Could you check a few things on this model? Use its own coordinates, in mm. Face numbers are marked on the shaded views. Coordinates: 2 decimals unless noted, no trailing zeros. Order: outer loops, then holes, each group sorted by start corner. A loop starts at its lowest first (then second) coordinate and runs counter-clockwise, first axis right, second up. Notation, with made-up numbers: (18.25, 8) -> (29.25, 8) arc R20 cw to (29.25, 38) -> close; hole circle Ø9 at (22, 67.25). An arc over 180 degrees is marked (long way). Put each result on its own line as item: value. Start each with the question number.
Q1. If we section it at A-A (y = -12): Count the separate pieces of the cut face and the enclosed holes in it, and give its area (3 significant figures).
Q2. If we section it at B-B (z = 5.75): Please give me the cut outline in (x, y), and give its area (3 significant figures).
Q3. Please list where these lines run through material, in increasing order: line 1 along Y through (x, z) = (-12, 6); line 2 along X through (y, z) = (-13, 4.5).
Q4. If we section it at C-C (x = -28): Please give me the cut outline in (y, z).
Q5. Will these pins go through, and if not, where does the flat tip stop? pin 1 (1 mm diameter, centred on x = -27, y = 2.5, fed in from -Z); pin 2 (3 mm diameter, centred on x = 24, z = 3.5, fed in from -Y).
Q6. We'd pull the mould along X, two halves only. Please class the marked faces 1, 2, 3 and 4: +X half, -X half, draft (parallel to the pull), parting line (faces both ways), or undercut.
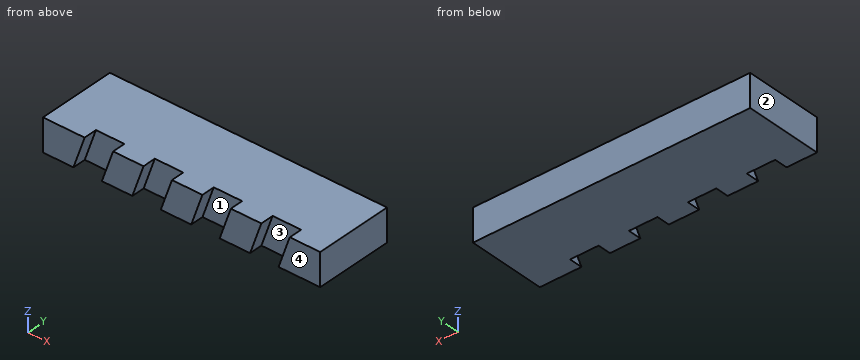
from build123d import *

# Parameters (mm, degrees)
F1_DEPTH = 10
F2_SIZE2 = 3.442485
F2_SIZE  = 9.99999
F3_SIZE2 = 3.442485
F3_SIZE  = 9.99999
F4_SIZE2 = 3.442485
F4_SIZE  = 9.99999
F5_SIZE2 = 3.442485
F5_SIZE  = 9.99999
F6_SIZE2 = 3.442485
F6_SIZE  = 9.99999
F7_SIZE2 = 3.442485
F7_SIZE  = 9.99999
F8_SIZE2 = 3.442485
F8_SIZE  = 9.99999
F9_SIZE2 = 3.442485
F9_SIZE  = 9.99999


# Not quite as in the source:
# - a fillet or chamfer is up to 0.001 mm smaller than in the source, because OpenCascade refuses the exact size


with BuildPart() as f1:
    # F0 (on Top) → F1 (new body)
    with BuildSketch(Plane.XY):
        Polygon((41.1003320895, 9.3217377585), (-44.0996679105, 9.3217377585), (-44.0996679105, -10.6782622415), (-44.0996679105, -14.7482622415), (-31.2996679105, -14.7482622415), (-31.2996679105, -10.6782622415), (-25.9996679105, -10.6782622415), (-25.9996679105, -14.7482622415), (-13.1996679105, -14.7482622415), (-13.1996679105, -10.6782622415), (-7.8996679105, -10.6782622415), (-7.8996679105, -14.7482622415), (4.9003320895, -14.7482622415), (4.9003320895, -10.6782622415), (10.2003320895, -10.6782622415), (10.2003320895, -14.7482622415), (23.0003320895, -14.7482622415), (23.0003320895, -10.6782622415), (28.3003320895, -10.6782622415), (28.3003320895, -14.7482622415), (41.1003320895, -14.7482622415), (41.1003320895, -10.6782622415), align=None)
    extrude(amount=F1_DEPTH)

    # F2 (size 10 and 3.4424952484 in the source; OpenCascade refuses exactly that, so slightly less here)
    f2_edges = [f1.edges().sort_by_distance(p)[0] for p in [
        (-31.299668, -12.713262, 0),
    ]]
    f2_side = f1.faces().sort_by_distance((-31.299668, -12.713262, 5))[0]
    chamfer(f2_edges, length=F2_SIZE, length2=F2_SIZE2, reference=f2_side)

    # F3 (size 10 and 3.4424952484 in the source; OpenCascade refuses exactly that, so slightly less here)
    f3_edges = [f1.edges().sort_by_distance(p)[0] for p in [
        (-25.999668, -12.713262, 10),
    ]]
    f3_side = f1.faces().sort_by_distance((-25.999668, -12.713262, 5))[0]
    chamfer(f3_edges, length=F3_SIZE, length2=F3_SIZE2, reference=f3_side)

    # F4 (size 10 and 3.4424952484 in the source; OpenCascade refuses exactly that, so slightly less here)
    f4_edges = [f1.edges().sort_by_distance(p)[0] for p in [
        (-13.199668, -12.713262, 0),
    ]]
    f4_side = f1.faces().sort_by_distance((-13.199668, -12.713262, 5))[0]
    chamfer(f4_edges, length=F4_SIZE, length2=F4_SIZE2, reference=f4_side)

    # F5 (size 10 and 3.4424952484 in the source; OpenCascade refuses exactly that, so slightly less here)
    f5_edges = [f1.edges().sort_by_distance(p)[0] for p in [
        (-7.899668, -12.713262, 10),
    ]]
    f5_side = f1.faces().sort_by_distance((-7.899668, -12.713262, 5))[0]
    chamfer(f5_edges, length=F5_SIZE, length2=F5_SIZE2, reference=f5_side)

    # F6 (size 10 and 3.4424952484 in the source; OpenCascade refuses exactly that, so slightly less here)
    f6_edges = [f1.edges().sort_by_distance(p)[0] for p in [
        (4.900332, -12.713262, 0),
    ]]
    f6_side = f1.faces().sort_by_distance((4.900332, -12.713262, 5))[0]
    chamfer(f6_edges, length=F6_SIZE, length2=F6_SIZE2, reference=f6_side)

    # F7 (size 10 and 3.4424952484 in the source; OpenCascade refuses exactly that, so slightly less here)
    f7_edges = [f1.edges().sort_by_distance(p)[0] for p in [
        (10.200332, -12.713262, 10),
    ]]
    f7_side = f1.faces().sort_by_distance((10.200332, -12.713262, 5))[0]
    chamfer(f7_edges, length=F7_SIZE, length2=F7_SIZE2, reference=f7_side)

    # F8 (size 10 and 3.4424952484 in the source; OpenCascade refuses exactly that, so slightly less here)
    f8_edges = [f1.edges().sort_by_distance(p)[0] for p in [
        (23.000332, -12.713262, 0),
    ]]
    f8_side = f1.faces().sort_by_distance((23.000332, -12.713262, 5))[0]
    chamfer(f8_edges, length=F8_SIZE, length2=F8_SIZE2, reference=f8_side)

    # F9 (size 10 and 3.4424952484 in the source; OpenCascade refuses exactly that, so slightly less here)
    f9_edges = [f1.edges().sort_by_distance(p)[0] for p in [
        (28.300332, -12.713262, 10),
    ]]
    f9_side = f1.faces().sort_by_distance((28.300332, -12.713262, 5))[0]
    chamfer(f9_edges, length=F9_SIZE, length2=F9_SIZE2, reference=f9_side)


solid = f1.part
The answers:
1. separate pieces: 5
1. enclosed holes: 0
1. area: 502 mm^2
2. outline: (-44.1, -14.75) -> (-32.76, -14.75) -> (-32.76, -10.68) -> (-24.02, -10.68) -> (-24.02, -14.75) -> (-14.66, -14.75) -> (-14.66, -10.68) -> (-5.92, -10.68) -> (-5.92, -14.75) -> (3.44, -14.75) -> (3.44, -10.68) -> (12.18, -10.68) -> (12.18, -14.75) -> (21.54, -14.75) -> (21.54, -10.68) -> (30.28, -10.68) -> (30.28, -14.75) -> (41.1, -14.75) -> (41.1, 9.32) -> (-44.1, 9.32) -> close
2. area: 1,910 mm^2
3. line 1: -10.68 to 9.32
3. line 2: -44.1 to -33.19, -24.45 to -15.09, -6.35 to 3.01, 11.75 to 21.11, 29.85 to 41.1
4. outline: (-10.68, 0) -> (9.32, 0) -> (9.32, 10) -> (-10.68, 10) -> close
5. pin 1: z = 0
5. pin 2: y = -10.68
6. face 1: undercut
6. face 2: -X half
6. face 3: undercut
6. face 4: draft
